```python
from build123d import *

# Parameters (mm, degrees)
SKETCH1_W           = 50.8
SKETCH1_H           = 50.8
SKETCH1_W_2         = 31.75
SKETCH1_H_2         = 31.75
BOSS_EXTRUDE1_DEPTH = 6.35
SKETCH2_W           = 50.8
SKETCH2_H           = 6.35
BOSS_EXTRUDE2_DEPTH = 25.4
FILLET1_R           = 6.35
SKETCH3_R           = 3.175
CUT_EXTRUDE1_DEPTH  = 58.15


with BuildPart() as part:
    # Sketch1 → Boss-Extrude1 (new, symmetric)
    with BuildSketch(Plane(origin=(0, 0, 0), x_dir=(0, 0, -1), z_dir=(1, 0, 0))):
        Rectangle(SKETCH1_W, SKETCH1_H)
        Rectangle(SKETCH1_W_2, SKETCH1_H_2, mode=Mode.SUBTRACT)
    extrude(amount=BOSS_EXTRUDE1_DEPTH, both=True)

    # Sketch2 → Boss-Extrude2 (add, symmetric)
    with BuildSketch(Plane(origin=(0, 0, 0), x_dir=(0, 0, -1), z_dir=(1, 0, 0))):
        with Locations((0, -22.225)):
            Rectangle(SKETCH2_W, SKETCH2_H)
    extrude(amount=BOSS_EXTRUDE2_DEPTH, both=True)

    # Fillet1
    # the kernel refuses this fillet: 6.35 mm, written as the material it adds along each edge
    with BuildSketch(Plane(origin=(-6.35, -19.05, -25.4), x_dir=(0, 1, 0), z_dir=(0, 0, 1))) as fillet1_piece_1_section:
        with BuildLine():
            CenterArc((FILLET1_R, FILLET1_R), FILLET1_R, 180, 90)
            Line((0, FILLET1_R), (0, 0))
            Line((0, 0), (FILLET1_R, 0))
        make_face()
    fillet1_piece_1 = extrude(amount=50.8, mode=Mode.PRIVATE)
    fillet1_piece_1 = split(fillet1_piece_1, bisect_by=Plane(origin=(-6.502453224, -14.838357518, -15.875), z_dir=(0, 0, -1)), keep=Keep.TOP, mode=Mode.PRIVATE)
    fillet1_piece_1 = split(fillet1_piece_1, bisect_by=Plane(origin=(-6.502453224, -15.875, -20.6375), z_dir=(0, 1, 0)), keep=Keep.TOP, mode=Mode.PRIVATE)
    add(fillet1_piece_1)
    with BuildSketch(Plane(origin=(-6.35, -19.05, -25.4), x_dir=(0, 1, 0), z_dir=(0, 0, 1))) as fillet1_piece_2_section:
        with BuildLine():
            CenterArc((FILLET1_R, FILLET1_R), FILLET1_R, 180, 90)
            Line((0, FILLET1_R), (0, 0))
            Line((0, 0), (FILLET1_R, 0))
        make_face()
    fillet1_piece_2 = extrude(amount=50.8, mode=Mode.PRIVATE)
    fillet1_piece_2 = split(fillet1_piece_2, bisect_by=Plane(origin=(-7.970012381, -18.006112297, -15.875), z_dir=(0, 0, -1)), keep=Keep.TOP, mode=Mode.PRIVATE)
    fillet1_piece_2 = split(fillet1_piece_2, bisect_by=Plane(origin=(-7.970012381, -15.875, -20.6375), z_dir=(0, -1, 0)), keep=Keep.TOP, mode=Mode.PRIVATE)
    add(fillet1_piece_2)
    with BuildSketch(Plane(origin=(-6.35, -19.05, -25.4), x_dir=(0, 1, 0), z_dir=(0, 0, 1))) as fillet1_piece_3_section:
        with BuildLine():
            CenterArc((FILLET1_R, FILLET1_R), FILLET1_R, 180, 90)
            Line((0, FILLET1_R), (0, 0))
            Line((0, 0), (FILLET1_R, 0))
        make_face()
    fillet1_piece_3 = extrude(amount=50.8, mode=Mode.PRIVATE)
    fillet1_piece_3 = split(fillet1_piece_3, bisect_by=Plane(origin=(-7.970012381, -18.006112297, -15.875), z_dir=(0, 0, 1)), keep=Keep.TOP, mode=Mode.PRIVATE)
    fillet1_piece_3 = split(fillet1_piece_3, bisect_by=Plane(origin=(-7.970012381, -15.875, 0), z_dir=(0, -1, 0)), keep=Keep.TOP, mode=Mode.PRIVATE)
    fillet1_piece_3 = split(fillet1_piece_3, bisect_by=Plane(origin=(-7.970012381, -18.006112297, 15.875), z_dir=(0, 0, -1)), keep=Keep.TOP, mode=Mode.PRIVATE)
    add(fillet1_piece_3)
    with BuildSketch(Plane(origin=(-6.35, -19.05, -25.4), x_dir=(0, 1, 0), z_dir=(0, 0, 1))) as fillet1_piece_4_section:
        with BuildLine():
            CenterArc((FILLET1_R, FILLET1_R), FILLET1_R, 180, 90)
            Line((0, FILLET1_R), (0, 0))
            Line((0, 0), (FILLET1_R, 0))
        make_face()
    fillet1_piece_4 = extrude(amount=50.8, mode=Mode.PRIVATE)
    fillet1_piece_4 = split(fillet1_piece_4, bisect_by=Plane(origin=(-6.502453224, -15.875, 20.6375), z_dir=(0, 1, 0)), keep=Keep.TOP, mode=Mode.PRIVATE)
    fillet1_piece_4 = split(fillet1_piece_4, bisect_by=Plane(origin=(-6.502453224, -14.838357518, 15.875), z_dir=(0, 0, 1)), keep=Keep.TOP, mode=Mode.PRIVATE)
    add(fillet1_piece_4)
    with BuildSketch(Plane(origin=(-6.35, -19.05, -25.4), x_dir=(0, 1, 0), z_dir=(0, 0, 1))) as fillet1_piece_5_section:
        with BuildLine():
            CenterArc((FILLET1_R, FILLET1_R), FILLET1_R, 180, 90)
            Line((0, FILLET1_R), (0, 0))
            Line((0, 0), (FILLET1_R, 0))
        make_face()
    fillet1_piece_5 = extrude(amount=50.8, mode=Mode.PRIVATE)
    fillet1_piece_5 = split(fillet1_piece_5, bisect_by=Plane(origin=(-7.970012381, -15.875, 20.6375), z_dir=(0, -1, 0)), keep=Keep.TOP, mode=Mode.PRIVATE)
    fillet1_piece_5 = split(fillet1_piece_5, bisect_by=Plane(origin=(-7.970012381, -18.006112297, 15.875), z_dir=(0, 0, 1)), keep=Keep.TOP, mode=Mode.PRIVATE)
    add(fillet1_piece_5)
    with BuildSketch(Plane(origin=(6.35, -19.05, -25.4), x_dir=(1, 0, 0), z_dir=(0, 0, 1))) as fillet1_piece_6_section:
        with BuildLine():
            CenterArc((FILLET1_R, FILLET1_R), FILLET1_R, 180, 90)
            Line((0, FILLET1_R), (0, 0))
            Line((0, 0), (FILLET1_R, 0))
        make_face()
    fillet1_piece_6 = extrude(amount=50.8, mode=Mode.PRIVATE)
    fillet1_piece_6 = split(fillet1_piece_6, bisect_by=Plane(origin=(7.970012381, -15.875, -20.6375), z_dir=(0, -1, 0)), keep=Keep.TOP, mode=Mode.PRIVATE)
    fillet1_piece_6 = split(fillet1_piece_6, bisect_by=Plane(origin=(7.970012381, -18.006112297, -15.875), z_dir=(0, 0, -1)), keep=Keep.TOP, mode=Mode.PRIVATE)
    add(fillet1_piece_6)
    with BuildSketch(Plane(origin=(6.35, -19.05, -25.4), x_dir=(1, 0, 0), z_dir=(0, 0, 1))) as fillet1_piece_7_section:
        with BuildLine():
            CenterArc((FILLET1_R, FILLET1_R), FILLET1_R, 180, 90)
            Line((0, FILLET1_R), (0, 0))
            Line((0, 0), (FILLET1_R, 0))
        make_face()
    fillet1_piece_7 = extrude(amount=50.8, mode=Mode.PRIVATE)
    fillet1_piece_7 = split(fillet1_piece_7, bisect_by=Plane(origin=(6.502453224, -15.875, -20.6375), z_dir=(0, 1, 0)), keep=Keep.TOP, mode=Mode.PRIVATE)
    fillet1_piece_7 = split(fillet1_piece_7, bisect_by=Plane(origin=(6.502453224, -14.838357518, -15.875), z_dir=(0, 0, -1)), keep=Keep.TOP, mode=Mode.PRIVATE)
    add(fillet1_piece_7)
    with BuildSketch(Plane(origin=(6.35, -19.05, -25.4), x_dir=(1, 0, 0), z_dir=(0, 0, 1))) as fillet1_piece_8_section:
        with BuildLine():
            CenterArc((FILLET1_R, FILLET1_R), FILLET1_R, 180, 90)
            Line((0, FILLET1_R), (0, 0))
            Line((0, 0), (FILLET1_R, 0))
        make_face()
    fillet1_piece_8 = extrude(amount=50.8, mode=Mode.PRIVATE)
    fillet1_piece_8 = split(fillet1_piece_8, bisect_by=Plane(origin=(7.970012381, -18.006112297, 15.875), z_dir=(0, 0, -1)), keep=Keep.TOP, mode=Mode.PRIVATE)
    fillet1_piece_8 = split(fillet1_piece_8, bisect_by=Plane(origin=(7.970012381, -15.875, 0), z_dir=(0, -1, 0)), keep=Keep.TOP, mode=Mode.PRIVATE)
    fillet1_piece_8 = split(fillet1_piece_8, bisect_by=Plane(origin=(7.970012381, -18.006112297, -15.875), z_dir=(0, 0, 1)), keep=Keep.TOP, mode=Mode.PRIVATE)
    add(fillet1_piece_8)
    with BuildSketch(Plane(origin=(6.35, -19.05, -25.4), x_dir=(1, 0, 0), z_dir=(0, 0, 1))) as fillet1_piece_9_section:
        with BuildLine():
            CenterArc((FILLET1_R, FILLET1_R), FILLET1_R, 180, 90)
            Line((0, FILLET1_R), (0, 0))
            Line((0, 0), (FILLET1_R, 0))
        make_face()
    fillet1_piece_9 = extrude(amount=50.8, mode=Mode.PRIVATE)
    fillet1_piece_9 = split(fillet1_piece_9, bisect_by=Plane(origin=(7.970012381, -18.006112297, 15.875), z_dir=(0, 0, 1)), keep=Keep.TOP, mode=Mode.PRIVATE)
    fillet1_piece_9 = split(fillet1_piece_9, bisect_by=Plane(origin=(7.970012381, -15.875, 20.6375), z_dir=(0, -1, 0)), keep=Keep.TOP, mode=Mode.PRIVATE)
    add(fillet1_piece_9)
    with BuildSketch(Plane(origin=(6.35, -19.05, -25.4), x_dir=(1, 0, 0), z_dir=(0, 0, 1))) as fillet1_piece_10_section:
        with BuildLine():
            CenterArc((FILLET1_R, FILLET1_R), FILLET1_R, 180, 90)
            Line((0, FILLET1_R), (0, 0))
            Line((0, 0), (FILLET1_R, 0))
        make_face()
    fillet1_piece_10 = extrude(amount=50.8, mode=Mode.PRIVATE)
    fillet1_piece_10 = split(fillet1_piece_10, bisect_by=Plane(origin=(6.502453224, -14.838357518, 15.875), z_dir=(0, 0, 1)), keep=Keep.TOP, mode=Mode.PRIVATE)
    fillet1_piece_10 = split(fillet1_piece_10, bisect_by=Plane(origin=(6.502453224, -15.875, 20.6375), z_dir=(0, 1, 0)), keep=Keep.TOP, mode=Mode.PRIVATE)
    add(fillet1_piece_10)

    # Sketch3 → Cut-Extrude1 (cut, through all)
    with BuildSketch(Plane(origin=(0, -19.05, 0), x_dir=(1, 0, 0), z_dir=(0, 1, 0))):
        with Locations(Location((19.05, 0, 0), (0, 0, 270))):
            Circle(SKETCH3_R)
    cut_extrude1 = extrude(amount=-CUT_EXTRUDE1_DEPTH, mode=Mode.SUBTRACT)

    # Mirror1: Cut-Extrude1 across plane
    add(cut_extrude1.mirror(Plane(origin=(0, 0, 0), x_dir=(0, 0, 1), z_dir=(1, 0, 0))), mode=Mode.SUBTRACT)


solid = part.part
```
Can you work these out from the model? Positions are in its coordinate system, mm. A direction names the side the tool comes from. Give positions to 0.01 mm unless a question says otherwise; leave off trailing zeros. Loops run counter-clockwise (first coordinate to the right, second up) from the corner with the lowest first, then second, coordinate; pieces in that order, holes last. Notation, with made-up numbers: M -34,-28.75 L 0,-28.75 A16 ccw 0,0.25 Z; hole C 89,85 d10. An arc over 180 degrees is marked long. One line per question, with ' | ' between items. Start each with the question number.
Q1. If we section it at D-D (z = 0): Please give me the cut outline in (x, y) (3 decimals), plus the area to 3 significant figures.
Q2. For pin 1 Ø19 at (y, z) = (9.5, -4) entering from +X; pin 2 Ø4 at (y, z) = (-16, 0.5) entering from -X; pin 3 Ø14 at (x, z) = (17.5, 2.5) entering from +Y, each with a flat end and sliding along its axis, tell me the tip position at first contact or that it passes through.
Q3. If we mould it in two halves opening along Z, with no side actions, what happens to faces 4 (the flat face through (0, 0, 15.875)), 5 (the flat face through (0, 0, -15.875)), 6 (the flat face through (-6.35, 19, 0)), 7 (the flat face through (0, -5, 25.4))? For each: +Z half, -Z half, draft (parallel to the pull), parting line (faces both ways), or undercut.
Q4. For faces 1 (the flat face through (-23, -19.05, 0)), 2 (the flat face through (0, 15.875, 0)), 3 (the flat face through (6.35, 19, 0)), which set-ups out of +Z, -Z, +X, -X, +Y, -Y let a thin tool reach every point of the face, with its end or its side?
Q5. If we section it at A-A (y = 5.5): Please give me the cut outline in (x, z) (3 decimals).
Q6. If we section it at B-B (x = 19.05): Please give me the cut outline in (y, z) (3 decimals).
Q7. If we section it at C-C (z = 14): Please give me the cut outline in (x, y) (3 decimals), plus the area to 3 significant figures.
Q8. If I drill on line 1 (X direction, y = -23.25, z = 0) (3 decimals); line 2 (Z direction, x = 19, y = -22); line 3 (Z direction, x = 3, y = 12.5) (3 decimals), over which ranges is the centre line in solid material (lowest first)? Write a range as from..to.
Computed:
1) outline: M -25.4,-25.4 L -22.225,-25.4 L -22.225,-19.05 L -25.4,-19.05 Z; M -15.875,-25.4 L 15.875,-25.4 L 15.875,-19.05 L 12.7,-19.05 A6.35 cw 7.201,-15.875 L -7.201,-15.875 A6.35 cw -12.7,-19.05 L -15.875,-19.05 Z; M -6.35,15.875 L 6.35,15.875 L 6.35,25.4 L -6.35,25.4 Z; M 22.225,-25.4 L 25.4,-25.4 L 25.4,-19.05 L 22.225,-19.05 Z | area: 419 mm²
2) pin 1: stops at x = 6.35 | pin 2: stops at x = -9.2 | pin 3: stops at y = -18.66
3) face 4: undercut | face 5: undercut | face 6: draft | face 7: +Z half
4) face 1: +Z, -Z, -X, +Y | face 2: +X, -X | face 3: +Z, -Z, +X, +Y
5) outline: M -6.35,-25.4 L 6.35,-25.4 L 6.35,-15.875 L -6.35,-15.875 Z; M -6.35,15.875 L 6.35,15.875 L 6.35,25.4 L -6.35,25.4 Z
6) outline: M -25.4,-25.4 L -19.05,-25.4 L -19.05,-3.175 L -25.4,-3.175 Z; M -25.4,3.175 L -19.05,3.175 L -19.05,25.4 L -25.4,25.4 Z
7) outline: M -25.4,-25.4 L 25.4,-25.4 L 25.4,-19.05 L 12.7,-19.05 A6.35 cw 7.201,-15.875 L -7.201,-15.875 A6.35 cw -12.7,-19.05 L -25.4,-19.05 Z; M -6.35,15.875 L 6.35,15.875 L 6.35,25.4 L -6.35,25.4 Z | area: 499 mm²
8) line 1: x = -25.4..-22.225, -15.875..15.875, 22.225..25.4 | line 2: z = -25.4..-3.17, 3.17..25.4 | line 3: z = -25.4..-15.875, 15.875..25.4
